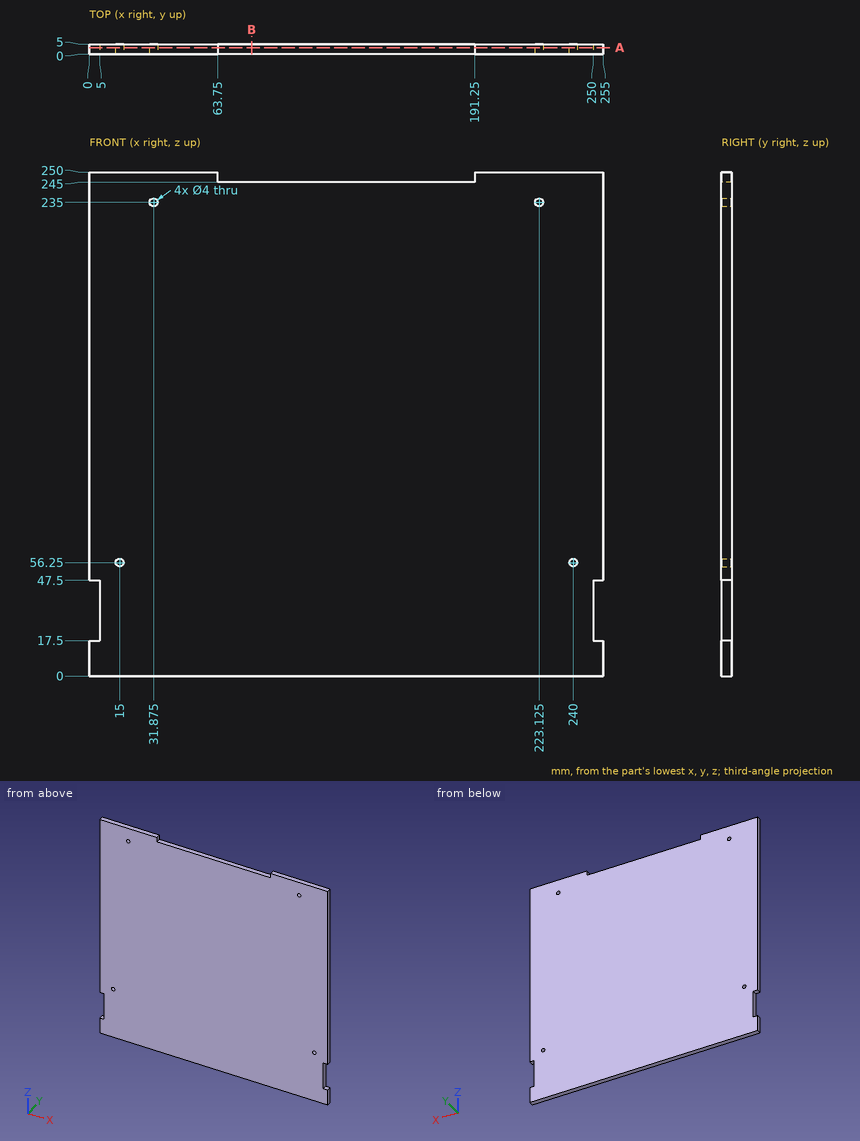
Verification items for this drawing (mm, ordinates from the low corner). Give positions to 0.01 mm unless a question says otherwise; leave off trailing zeros. Write each loop counter-clockwise with the first axis right and the second up, starting at its lowest first coordinate (ties: lowest second). Pieces come first, ordered by that corner, then holes. Notation, with made-up numbers: (24.5, 78.25) -> (81.5, 78.25) arc R11 cw to (81.5, 96.25) -> close; hole circle Ø6 at (-35, 78). An arc over 180 degrees is marked (long way). Use CSV: the item, a comma, the result in double quotes.
(1) Material ranges on L1, parallel to X at y = 2.4, z = 56.25; L2, parallel to X at y = 3.3, z = 235 (3 decimals); L3, parallel to Z at x = 240, y = 2.9, recorded low to high.
Derived:
L1,"x = 0 to 13, 17 to 238, 242 to 255"
L2,"x = 0 to 29.875, 33.875 to 221.125, 225.125 to 255"
L3,"z = 0 to 54.25, 58.25 to 250"
(2) Sectioned sample at B-B (x = 80.5). Record the cut outline in (y, z).
Derived:
outline,"(0, 0) -> (5, 0) -> (5, 245) -> (0, 245) -> close"
(3) Sectioned sample at A-A (y = 3.2). Record the cut outline in (x, z) (3 decimals).
Derived:
outline,"(0, 0) -> (255, 0) -> (255, 17.5) -> (250, 17.5) -> (250, 47.5) -> (255, 47.5) -> (255, 250) -> (191.25, 250) -> (191.25, 245) -> (63.75, 245) -> (63.75, 250) -> (0, 250) -> (0, 47.5) -> (5, 47.5) -> (5, 17.5) -> (0, 17.5) -> close; hole circle Ø4 at (15, 56.25); hole circle Ø4 at (31.875, 235); hole circle Ø4 at (223.125, 235); hole circle Ø4 at (240, 56.25)"
(4) Go/stop test with a flat-tipped pin: pin 1 (2.5 mm diameter, centred on y = 2, z = 37, fed in from +X). Record where the tip stops, or that it passes through.
Derived:
pin 1,"stops at x = 250"
